from build123d import *

# Parameters (mm, degrees)
SKETCH1_W           = 8.1
SKETCH1_H           = 12.3
BOSS_EXTRUDE1_DEPTH = 7
SKETCH2_R           = 3
BOSS_EXTRUDE2_DEPTH = 4
SKETCH3_R           = 1.8
CUT_EXTRUDE1_DEPTH  = 14
CHAMFER1_SIZE       = 0.3
SKETCH4_W           = 1.5
SKETCH4_H           = 0.5
BOSS_EXTRUDE3_DEPTH = 3.5


with BuildPart() as part:
    # Sketch1 → Boss-Extrude1 (new, symmetric)
    with BuildSketch(Plane.XY):
        Rectangle(SKETCH1_W, SKETCH1_H)
    extrude(amount=BOSS_EXTRUDE1_DEPTH, both=True)

    # Sketch2 → Boss-Extrude2 (add)
    with BuildSketch(Plane.XY.offset(7)):
        with Locations(Location((-0.85, 0.85, 0), (0, 0, 180))):
            Circle(SKETCH2_R)
    extrude(amount=BOSS_EXTRUDE2_DEPTH)

    # Sketch3 → Cut-Extrude1 (cut)
    with BuildSketch(Plane.XY.offset(11)):
        with Locations((-0.85, 0.85)):
            Circle(SKETCH3_R)
    extrude(amount=-CUT_EXTRUDE1_DEPTH, mode=Mode.SUBTRACT)

    # Chamfer1
    chamfer1_edges = [part.edges().sort_by_distance(p)[0] for p in [
        (-2.65, 0.85, 11),
    ]]
    chamfer(chamfer1_edges, length=CHAMFER1_SIZE)

    # Sketch4 → Boss-Extrude3 (add)
    with BuildSketch(Plane.XZ.offset(6.15)):
        with Locations((0.9, 6)):
            Rectangle(SKETCH4_W, SKETCH4_H)
        with Locations((-1.1, 2.3)):
            Rectangle(SKETCH4_W, SKETCH4_H)
        with Locations((0.9, 0.4)):
            Rectangle(SKETCH4_W, SKETCH4_H)
        with Locations((-1.1, -3.3)):
            Rectangle(SKETCH4_W, SKETCH4_H)
        with Locations((0.9, -5.8)):
            Rectangle(SKETCH4_W, SKETCH4_H)
    extrude(amount=BOSS_EXTRUDE3_DEPTH)


solid = part.part
Can you work these out from the model? Positions are in its coordinate system, mm. A direction names the side the tool comes from. Coordinates: 2 decimals unless noted, no trailing zeros. Write each loop counter-clockwise with the first axis right and the second up, starting at its lowest first coordinate (ties: lowest second). Pieces come first, ordered by that corner, then holes. Notation, with made-up numbers: (10, 1) -> (60, 1) arc R8 ccw to (60, 7) -> close; hole circle Ø11 at (40.5, -7.75). An arc over 180 degrees is marked (long way). Write each question's results on one line, items separated by ' | '. Start each with the question number.
Item 1: On a 3-axis mill with a long thin cutter (end or side, diameter ignored), from which of +Z, -Z, +X, -X, +Y, -Y can I reach the whole of each face in a straight line? I mean faces 5 (the flat face through (1, -8, 0.65)), 6 (the flat face through (-2, 3, 11)), 7 (the flat face through (1, -8, 6.25)), 8 (the flat face through (-1, -8, -3.55)), 9 (the flat face through (-4.05, 0, 0)). Say none if no direction works.
Item 2: Thinking about a two-plate mould opening in Y: for faces 1 (the cylindrical face through (-1.084, 2.635, 3.946)), 2 (the flat face through (-1, 1, -3)), 3 (the flat face through (0, 0, -7)), 4 (the cylindrical face through (2.147, 0.718, 8.972)), which applies, released by +Y, released by -Y, zero draft, split by the parting line, or undercut?
Item 3: If we section it at C-C, the plane z = 3: Write out the boundary of the cut face in (x, y), and give its area (3 significant figures).
Item 4: Please list where these lines run through material, in increasing order: probe 1 along Y at (x, z) = (-0.85, 7.5); probe 2 along Y at (x, z) = (-0.85, 4.75); probe 3 along Z at (x, y) = (2.5, 4).
Item 5: If we section it at A-A, the plane y = -7.75: Write out the boundary of the cut face in (x, z).
Item 6: I'm going to push flat-ended pins straight in: P1, Ø1.6, axis at x = -1, y = -8.5, coming from the -Z side; P2, Ø1.6, axis at x = 1, y = -7.5, coming from the +Z side; P3, Ø1.2, axis at x = -0.5, y = -7.5, coming from the +Z side. Where does each tip first touch, or does it pass through?
Item 7: If we section it at B-B, the plane x = -0.85: Write out the boundary of the cut face in (y, z).
Item 8: If we section it at D-D, the plane y = 0.85: Write out the boundary of the cut face in (x, z), and give its area (3 significant figures).
Answer block:
1) face 5: +X, -X, -Y | face 6: +Z, +X, -X, +Y, -Y | face 7: +Z, +X, -X, -Y | face 8: -Z, +X, -X, -Y | face 9: +Z, -Z, -X, +Y, -Y
2) face 1: undercut | face 2: undercut | face 3: zero draft | face 4: split by the parting line
3) outline: (-4.05, -6.15) -> (4.05, -6.15) -> (4.05, 6.15) -> (-4.05, 6.15) -> close; hole circle Ø3.6 at (-0.85, 0.85) | area: 89.5 mm²
4) probe 1: -2.15 to -0.95, 2.65 to 3.85 | probe 2: -6.15 to -0.95, 2.65 to 6.15 | probe 3: -7 to 7
5) outline: (-1.85, -3.55) -> (-0.35, -3.55) -> (-0.35, -3.05) -> (-1.85, -3.05) -> close; (-1.85, 2.05) -> (-0.35, 2.05) -> (-0.35, 2.55) -> (-1.85, 2.55) -> close; (0.15, -6.05) -> (1.65, -6.05) -> (1.65, -5.55) -> (0.15, -5.55) -> close; (0.15, 0.15) -> (1.65, 0.15) -> (1.65, 0.65) -> (0.15, 0.65) -> close; (0.15, 5.75) -> (1.65, 5.75) -> (1.65, 6.25) -> (0.15, 6.25) -> close
6) P1: z = -3.55 | P2: z = 6.25 | P3: z = 2.55
7) outline: (-9.65, -3.55) -> (-6.15, -3.55) -> (-6.15, -7) -> (6.15, -7) -> (6.15, 7) -> (3.85, 7) -> (3.85, 11) -> (2.95, 11) -> (2.65, 10.7) -> (2.65, -3) -> (-0.95, -3) -> (-0.95, 10.7) -> (-1.25, 11) -> (-2.15, 11) -> (-2.15, 7) -> (-6.15, 7) -> (-6.15, 2.55) -> (-9.65, 2.55) -> (-9.65, 2.05) -> (-6.15, 2.05) -> (-6.15, -3.05) -> (-9.65, -3.05) -> close
8) outline: (-4.05, -7) -> (4.05, -7) -> (4.05, 7) -> (2.15, 7) -> (2.15, 11) -> (1.25, 11) -> (0.95, 10.7) -> (0.95, -3) -> (-2.65, -3) -> (-2.65, 10.7) -> (-2.95, 11) -> (-3.85, 11) -> (-3.85, 7) -> (-4.05, 7) -> close | area: 86.9 mm²
